```python
from build123d import *

# Parameters (mm, degrees)
SKETCH1_R           = 6
BOSS_EXTRUDE1_DEPTH = 8
SKETCH2_R           = 5
BOSS_EXTRUDE2_DEPTH = 79
SKETCH3_R           = 3
BOSS_EXTRUDE3_DEPTH = 7
SKETCH4_R           = 3
CUT_EXTRUDE1_DEPTH  = 8.5


with BuildPart() as part:
    # Sketch1 → Boss-Extrude1 (new body, symmetric)
    with BuildSketch(Plane(origin=(0, 0, 0), x_dir=(1, 0, 0), z_dir=(0, 1, 0))):
        Circle(SKETCH1_R)
    extrude(amount=BOSS_EXTRUDE1_DEPTH, both=True)

    # Sketch2 → Boss-Extrude2 (add)
    with BuildSketch(Plane.XZ.offset(8)):
        Circle(SKETCH2_R)
    extrude(amount=BOSS_EXTRUDE2_DEPTH)

    # Sketch3 → Boss-Extrude3 (add)
    with BuildSketch(Plane.XZ.offset(87)):
        Circle(SKETCH3_R)
    extrude(amount=BOSS_EXTRUDE3_DEPTH)

    # Sketch4 → Cut-Extrude1 (cut, symmetric)
    with BuildSketch(Plane.XY):
        Circle(SKETCH4_R)
    extrude(amount=CUT_EXTRUDE1_DEPTH, both=True, mode=Mode.SUBTRACT)


solid = part.part
```
The model under review builds one solid part; all positions refer to its coordinate system, in mm. A direction names the side the tool comes from. Give positions to 0.01 mm unless a question says otherwise; leave off trailing zeros. Write each loop counter-clockwise with the first axis right and the second up, starting at its lowest first coordinate (ties: lowest second). Pieces come first, ordered by that corner, then holes.
(1) For P1, Ø4, axis at x = 1.5, y = -83, coming from the +Z side; P2, Ø5, axis at y = -80.5, z = 2, coming from the -X side; P3, Ø5.5, axis at x = 0, y = 0, coming from the -Z side; P4, Ø1.5, axis at x = -3.5, y = -40.5, coming from the -Z side, all flat-tipped, find the tip position at first contact; note any pin that passes through.
(2) Consider section A-A, the plane x = 0. Give the boundary of the cut face in (y, z), and give its area (3 significant figures).
(3) Tool access review of faces 1 (the flat face through (0, -94, 0)), 2 (the cylindrical face through (-1.08, -46.95, -4.88)): name each direction out of +Z, -Z, +X, -X, +Y, -Y from which nothing blocks a thin tool from reaching the whole face with its end or side.
(4) Consider section D-D, the plane y = -73.5. Give the boundary of the cut face in (x, z).
(5) Consider section B-B, the plane z = 0. Give the boundary of the cut face in (x, y).
(6) To check wall thickness, follow L1, parallel to Y at x = 0.25, z = -3.5; L2, parallel to Y at x = 0, z = -2.25; L3, parallel to Z at x = 4, y = -57.5. State the ranges of each line that lie inside material, in increasing order.
(7) Consider section C-C, the plane x = 4. Give the boundary of the cut face in (y, z).
Returned:
1. P1: stops at z = 5
1. P2: stops at x = -5
1. P3: passes through
1. P4: stops at z = -4.18
2. outline: (-94, -3) - (-87, -3) - (-87, -5) - (-8, -5) - (-8, -6) - (-3, -6) - (-3, 6) - (-8, 6) - (-8, 5) - (-87, 5) - (-87, 3) - (-94, 3) - close; (3, -6) - (8, -6) - (8, 6) - (3, 6) - close
2. area: 952 mm2
3. face 1: +Z, -Z, +X, -X, -Y
3. face 2: -Y
4. outline: circle Ø10 at (0, 0)
5. outline: (-6, -8) - (-5, -8) - (-5, -87) - (-3, -87) - (-3, -94) - (3, -94) - (3, -87) - (5, -87) - (5, -8) - (6, -8) - (6, 8) - (-6, 8) - close; hole circle Ø6 at (0, 0)
6. L1: y = -87 to -2.99, 2.99 to 8
6. L2: y = -94 to -3, 3 to 8
6. L3: z = -3 to 3
7. outline: (-87, -3) - (-8, -3) - (-8, -4.47) - (8, -4.47) - (8, 4.47) - (-8, 4.47) - (-8, 3) - (-87, 3) - close
